Can you work these out from the model? Positions are in its coordinate system, mm. Face numbers are marked on the shaded views. A direction names the side the tool comes from. Round coordinates to 2 decimals unless told otherwise and drop trailing zeros. Loops run counter-clockwise (first coordinate to the right, second up) from the corner with the lowest first, then second, coordinate; pieces in that order, holes last. Notation, with made-up numbers: (54.25, 29) -> (58.25, 29) arc R34 ccw to (58.25, 64) -> close; hole circle Ø2 at (46.25, 23). An arc over 180 degrees is marked (long way). Answer as a JSON object with one key per item and string values.
Autodesk Inventor part; units mm, degrees
ref_plane "YZ Plane" through (0, 0, 0) normal (1, 0, 0) x (0, 1, 0)
ref_plane "XZ Plane" through (0, 0, 0) normal (0, 1, 0) x (-1, 0, 0)
ref_plane "XY Plane" through (0, 0, 0) normal (0, 0, 1) x (1, 0, 0)
sketch "Sketch1" plane through (0, 0, 0) normal (0, 0, 1) x (1, 0, 0)
  line L0 (0, 0) -> (59, 0)
  line L1 (59, 0) -> (59, -25)
  line L2 (59, -25) -> (0, -25)
  line L3 (0, -25) -> (0, 0)
  dimension "d0" = 59
  dimension "d1" = 25
extrude "Extrusion1" add sketch "Sketch1" along normal blind 3
sketch "Sketch2" plane through (0, -25, 0) normal (-1, 0, 0) x (0, 0, 1)
  line L0 (3, 0) -> (3, 25)
  line L1 (3, 25) -> (-15, 25)
  line L2 (-15, 25) -> (-15, 0)
  line L3 (-15, 0) -> (3, 0)
  line L4 (3, 0) -> (3, 25)
  point P0 (0, 25)
  dimension "d4" = 18
extrude "Extrusion2" add sketch "Sketch2" along normal blind 3
properties part number "arduino array box v03 slot"
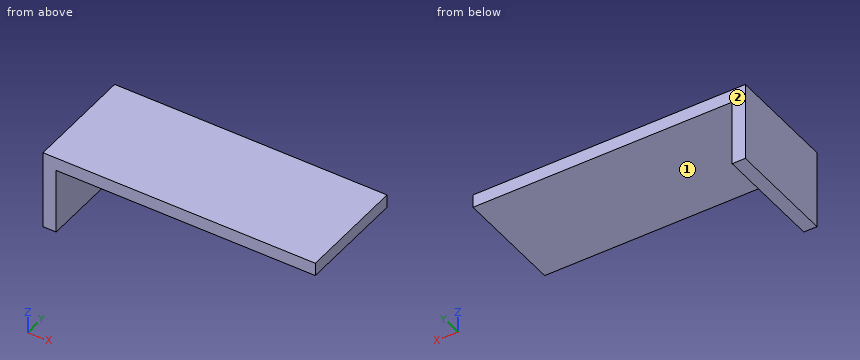
Q1. On a 3-axis mill with a long thin cutter (end or side, diameter ignored), from which of +Z, -Z, +X, -X, +Y, -Y can I reach the whole of each face in a straight line? I mean the marked faces 1 and 2. Say none if no direction works.
Determined:
{"face 1": "-Z, +X, +Y, -Y", "face 2": "+Z, -Z, +X, -X, +Y"}
Q2. I want a section at A-A, the plane y = -9.5. Write out the boundary of the cut face in (x, z).
Determined:
{"outline": "(-3, -15) -> (0, -15) -> (0, 0) -> (59, 0) -> (59, 3) -> (-3, 3) -> close"}
Q3. I'm going to push flat-ended pins straight in: pin 1 (1 mm diameter, centred on y = -10, z = -6.5, fed in from +X); pin 2 (1 mm diameter, centred on x = 7, y = -20, fed in from -Z). Where does each tip first touch, or does it pass through?
Determined:
{"pin 1": "x = 0", "pin 2": "z = 0"}
Q4. I want a section at C-C, the plane x = 18.5. Write out the boundary of the cut face in (y, z), then the cut area to 3 significant figures.
Determined:
{"outline": "(-25, 0) -> (0, 0) -> (0, 3) -> (-25, 3) -> close", "area": "75.0 mm²"}
Q5. If I drill on L1, parallel to Z at x = 48, y = -3; L2, parallel to X at y = -11.25, z = -11, over which ranges is the centre line in solid material (lowest first)? Write a range as [from, to].
Determined:
{"L1": "[0, 3]", "L2": "[-3, 0]"}
Q6. I want a section at B-B, the plane z = -8.25. Write out the boundary of the cut face in (x, y), then the cut area to 3 significant figures.
Determined:
{"outline": "(-3, -25) -> (0, -25) -> (0, 0) -> (-3, 0) -> close", "area": "75.0 mm²"}
